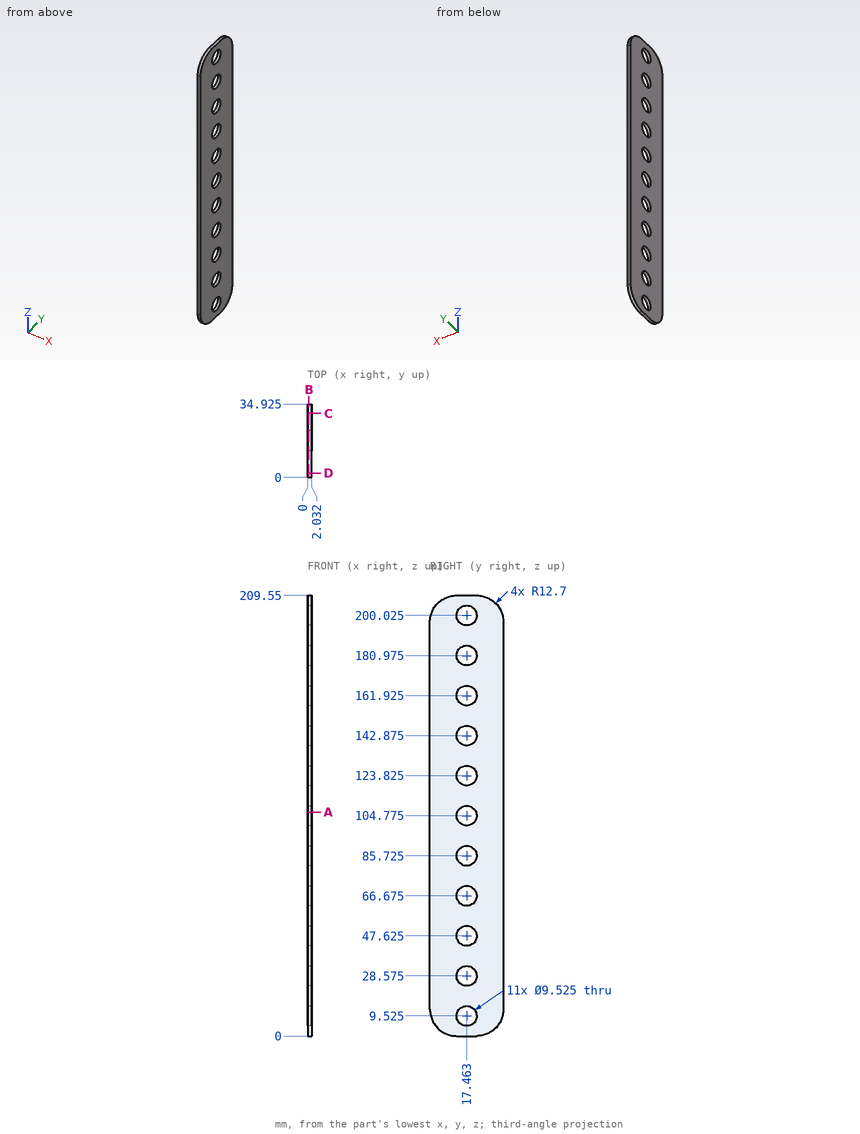
Could you check a few things on this drawing? It's one solid part, dimensions in mm from its lowest x, y, z. Round coordinates to 2 decimals unless told otherwise and drop trailing zeros. Order: outer loops, then holes, each group sorted by start corner. A loop starts at its lowest first (then second) coordinate and runs counter-clockwise, first axis right, second up. Notation, with made-up numbers: M 64,51.5 L 113,51.5 A13 cw 113,58.5 Z; hole C -7.5,20.25 d9. An arc over 180 degrees is marked long. One line per question, with ' | ' between items. Start each with the question number.
(1) Suppose I cut it at D-D on y = 2. List the corners of the cut face in (x, z) for me, then the cut area to 3 significant figures.
(2) Suppose I cut it at B-B on x = 0.6. Count the separate pieces of the cut face and the enclosed holes in it, then the cut area to 3 significant figures.
(3) Please list where these lines run through material, in increasing order: line 1 along Y through (x, z) = (0.85, 85.5) (1 decimal); line 2 along Z through (x, y) = (0.9, 23); line 3 along Y through (x, z) = (0.35, 126.5) (1 decimal).
(4) Suppose I cut it at A-A on z = 106.5. List the corners of the cut face in (x, y) for me (1 decimal).
(5) Suppose I cut it at C-C on y = 30.5. List the corners of the cut face in (x, z) for me (1 decimal).
Geometry results:
1) outline: M 0,5.86 L 2.03,5.86 L 2.03,203.69 L 0,203.69 Z | area: 402 mm²
2) separate pieces: 1 | enclosed holes: 11 | area: 6,400 mm²
3) line 1: 0 to 12.7, 22.2 to 34.9 | line 2: 0.02 to 209.53 | line 3: 0 to 13.5, 21.4 to 34.9
4) outline: M 0,0 L 2,0 L 2,13 L 0,13 Z; M 0,21.9 L 2,21.9 L 2,34.9 L 0,34.9 Z
5) outline: M 0,3.1 L 2,3.1 L 2,206.5 L 0,206.5 Z
